```python
from build123d import *

# Parameters (mm, degrees)
ESQUISSE1_R             = 50.8
BOSS_EXTRU_1_DEPTH      = 25
ESQUISSE2_R             = 25.4
ENL_V_MAT_EXTRU_1_DEPTH = 26
ESQUISSE3_R             = 42.5
ENL_V_MAT_EXTRU_2_DEPTH = 20
ESQUISSE4_R             = 2.5
ENL_V_MAT_EXTRU_3_DEPTH = 6
ESQUISSE5_R             = 2
ENL_V_MAT_EXTRU_4_DEPTH = 7.5


with BuildPart() as part:
    # Esquisse1 → Boss.-Extru.1 (new body)
    with BuildSketch(Plane.XY):
        Circle(ESQUISSE1_R)
    extrude(amount=BOSS_EXTRU_1_DEPTH)

    # Esquisse2 → Enlèv. mat.-Extru.1 (cut, through all)
    with BuildSketch(Plane.XY.offset(25)):
        Circle(ESQUISSE2_R)
    extrude(amount=-ENL_V_MAT_EXTRU_1_DEPTH, mode=Mode.SUBTRACT)

    # Esquisse3 → Enlèv. mat.-Extru.2 (cut)
    with BuildSketch(Plane(origin=(0, 0, 0), x_dir=(-1, 0, 0), z_dir=(0, 0, -1))):
        Circle(ESQUISSE3_R)
    extrude(amount=-ENL_V_MAT_EXTRU_2_DEPTH, mode=Mode.SUBTRACT)

    # Esquisse4 → Enlèv. mat.-Extru.3 (cut, through all)
    with BuildSketch(Plane(origin=(0, 0, 20), x_dir=(-1, 0, 0), z_dir=(0, 0, -1))):
        with Locations((-30.16, 0)):
            Circle(ESQUISSE4_R)
        with Locations((30.16, 0)):
            Circle(ESQUISSE4_R)
    extrude(amount=-ENL_V_MAT_EXTRU_3_DEPTH, mode=Mode.SUBTRACT)

    # Esquisse5 → Enlèv. mat.-Extru.4 (cut)
    with BuildSketch(Plane(origin=(0, 0, 0), x_dir=(-1, 0, 0), z_dir=(0, 0, -1))):
        with Locations((0, 46.647557519)):
            Circle(ESQUISSE5_R)
        with Locations((0, -47.352442481)):
            Circle(ESQUISSE5_R)
    extrude(amount=-ENL_V_MAT_EXTRU_4_DEPTH, mode=Mode.SUBTRACT)


solid = part.part
```
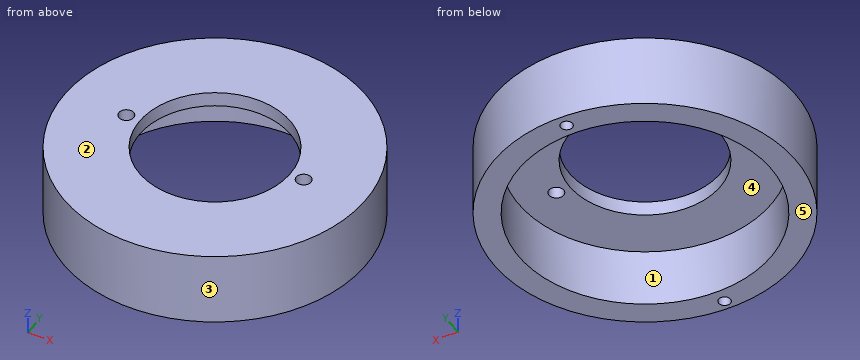
Source: CAD feature listing. Evaluate the final solid. Frame: model axes, mm. Face numbers are marked on the shaded views. A direction names the side the tool comes from. Coordinates: 2 decimals unless noted, no trailing zeros. Write each loop counter-clockwise with the first axis right and the second up, starting at its lowest first coordinate (ties: lowest second). Pieces come first, ordered by that corner, then holes. Notation, with made-up numbers: (-18.5, -7) - (25.5, -7) arc R21 cw to (25.5, 6) - close; hole circle Ø2 at (-3, -40). An arc over 180 degrees is marked (long way). Answer as a JSON object with one key per item and string values.
Q1. First-contact query: pin 1 Ø2.5 at (x, y) = (0, 46.65) entering from -Z; pin 2 Ø2 at (x, y) = (-10, 30) entering from -Z; pin 3 Ø2 at (y, z) = (-21.5, 3.5) entering from +X. Flat tips, straight axial feed; report the tip coordinate or a pass-through.
Ans:
{"pin 1": "stops at z = 7.5", "pin 2": "stops at z = 20", "pin 3": "stops at x = 46.48"}
Q2. Section query D-D, the plane z = 10. Output: boundary loops of the cut face in (x, y), plus the area to 3 significant figures.
Ans:
{"outline": "circle Ø101.6 at (0, 0); hole circle Ø85 at (0, 0)", "area": "2,430 mm2"}
Q3. Material intervals for line 1 (Y direction, x = 0, z = 4.5); line 2 (Y direction, x = 0, z = 21); line 3 (Y direction, x = -1, z = 15.75), sorted ascending. Write a range as [from, to].
Ans:
{"line 1": "y = [-50.8, -49.35], [-45.35, -42.5], [42.5, 44.65], [48.65, 50.8]", "line 2": "y = [-50.8, -25.4], [25.4, 50.8]", "line 3": "y = [-50.79, -42.49], [42.49, 50.79]"}
Q4. Set-up query: the marked faces 4 and 5. Return all of +Z, -Z, +X, -X, +Y, -Y with unobstructed straight access to the full face (end or side cutting, diameter ignored); none if empty.
Ans:
{"face 4": "-Z", "face 5": "-Z, +X, -X, +Y, -Y"}
Q5. Section query B-B, the plane y = -11. Output: boundary loops of the cut face in (x, z), plus the area to 3 significant figures.
Ans:
{"outline": "(-49.59, 0) - (-41.05, 0) - (-41.05, 20) - (-22.89, 20) - (-22.89, 25) - (-49.59, 25) - close; (22.89, 20) - (41.05, 20) - (41.05, 0) - (49.59, 0) - (49.59, 25) - (22.89, 25) - close", "area": "609 mm2"}
Q6. Section query C-C, the plane x = -5.5. Output: boundary loops of the cut face in (y, z), plus the area to 3 significant figures.
Ans:
{"outline": "(-50.5, 0) - (-42.14, 0) - (-42.14, 20) - (-24.8, 20) - (-24.8, 25) - (-50.5, 25) - close; (24.8, 20) - (42.14, 20) - (42.14, 0) - (50.5, 0) - (50.5, 25) - (24.8, 25) - close", "area": "591 mm2"}
Q7. Section query A-A, the plane y = 0. Output: boundary loops of the cut face in (x, z).
Ans:
{"outline": "(-50.8, 0) - (-42.5, 0) - (-42.5, 20) - (-32.66, 20) - (-32.66, 25) - (-50.8, 25) - close; (-27.66, 20) - (-25.4, 20) - (-25.4, 25) - (-27.66, 25) - close; (25.4, 20) - (27.66, 20) - (27.66, 25) - (25.4, 25) - close; (32.66, 20) - (42.5, 20) - (42.5, 0) - (50.8, 0) - (50.8, 25) - (32.66, 25) - close"}
Q8. Draft query along Y for the marked faces 1, 2 and 3. Return one class per face: released by +Y, released by -Y, zero draft, split by the parting line, or undercut.
Ans:
{"face 1": "undercut", "face 2": "zero draft", "face 3": "split by the parting line"}
